Design review of the part built by this model. Coordinates are the model's own, in mm. Give positions to 0.01 mm unless a question says otherwise; leave off trailing zeros. Write each loop counter-clockwise with the first axis right and the second up, starting at its lowest first coordinate (ties: lowest second). Pieces come first, ordered by that corner, then holes. Notation, with made-up numbers: M 42,44 L 49,44 A22 ccw 49,82 Z; hole C -5,-3.75 d2. An arc over 180 degrees is marked long. Answer in a Markdown table with one row per item.
```python
from build123d import *

# Parameters (mm, degrees)
F1_DEPTH = 127
F2_R     = 12.7


with BuildPart() as f1:
    # F0 (on Front) → F1 (new body)
    with BuildSketch(Plane.XZ):
        with BuildLine():
            Line((-63.5, 177.8), (-177.8, 177.8))
            Line((-177.8, 177.8), (-177.8, 0))
            Line((-177.8, 0), (0, 0))
            Line((0, 0), (0, 114.3))
            ThreePointArc((0, 114.3), (-18.598719, 159.201281), (-63.5, 177.8))
        make_face()
    extrude(amount=-F1_DEPTH)

    # F2
    f2_edges = [f1.edges().sort_by_distance(p)[0] for p in [
        (0, 63.5, 0),
    ]]
    fillet(f2_edges, radius=F2_R)


solid = f1.part
```
1) To check wall thickness, follow probe 1 along X at (y, z) = (121, 150); probe 2 along Z at (x, y) = (-16, 54); probe 3 along X at (y, z) = (116, 151.5). State the ranges of each line that lie inside material, in increasing order. Write a range as [from, to].
Geometry says:
| item | result |
|---|---|
| probe 1 | [-177.8, -10.99] |
| probe 2 | [0, 156.44] |
| probe 3 | [-177.8, -12.04] |
2) Add section A-A (y = 84). Write out the cut boundary in (x, z), and give its area (3 significant figures).
Geometry says:
| item | result |
|---|---|
| outline | M -177.8,0 L -12.7,0 A12.7 ccw 0,12.7 L 0,114.3 A63.5 ccw -63.5,177.8 L -177.8,177.8 Z |
| area | 30,700 mm^2 |
3) Add section B-B (z = 134.5). Write out the cut boundary in (x, y).
Geometry says:
| item | result |
|---|---|
| outline | M -177.8,0 L -3.3,0 L -3.3,127 L -177.8,127 Z |
4) The part is to be moulded in two halves that separate along Y. For faces 1 (the face through (-90, 0, 90)), 2 (the face through (-3.82, 64.39, 3.62)), 3 (the face through (-90, 127, 90)), say which applies: released by +Y, released by -Y, zero draft, split by the parting line, or undercut.
Geometry says:
| item | result |
|---|---|
| face 1 | released by -Y |
| face 2 | zero draft |
| face 3 | released by +Y |
5) Add section C-C (z = 161). Write out the cut boundary in (x, y), and give its area (3 significant figures).
Geometry says:
| item | result |
|---|---|
| outline | M -177.8,0 L -20.47,0 L -20.47,127 L -177.8,127 Z |
| area | 20,000 mm^2 |
6) Insertion check: P1, Ø10, axis at y = 63.5, z = 130, coming from the +X side; P2, Ø12, axis at x = -19.5, y = 80, coming from the +Z side. Each pin has a flat end and moves straight along its axis. Give the tip position at first contact, or say it passes through.
Geometry says:
| item | result |
|---|---|
| P1 | x = -0.91 |
| P2 | z = 165.17 |
